from build123d import *

# Parameters (mm, degrees)
F0_R             = 22.25
F1_DEPTH         = 0.8
F2_W             = 8
F2_H             = 8
F3_DEPTH         = 5.7
F4_W             = 8
F4_H             = 6
F5_DEPTH         = 2.9
F6_R             = 0.75
F7_DEPTH         = 0.8
F7_COPIES_COUNT  = 4
F7_COPIES_ANGLE  = 67.5
F7_COPIES1_COUNT = 4
F7_COPIES1_ANGLE = 337.5
F7_COPIES2_COUNT = 3
F7_COPIES2_ANGLE = 315
F7_COPIES3_COUNT = 3
F7_COPIES3_ANGLE = 225
F8_DEPTH         = 0.1
F8_COPIES_COUNT  = 4
F8_COPIES_ANGLE  = 67.5
F8_COPIES1_COUNT = 4
F8_COPIES1_ANGLE = 337.5
F8_COPIES2_COUNT = 3
F8_COPIES2_ANGLE = 315
F8_COPIES3_COUNT = 3
F8_COPIES3_ANGLE = 225


# Not quite as in the source:
# - after a boolean that leaves OpenCascade's solid faulty, fix() repairs it
# - a feature of the source that left no trace in its solid (it failed there, or was rolled back) is left out
# - a pattern or mirror of a feature is missing from the dataset's text; its kind, count and spacing are read off the source's solid


with BuildPart() as f1:
    # F0 (on Top) → F1 (new body)
    with BuildSketch(Plane.XY):
        Circle(F0_R)
    extrude(amount=F1_DEPTH)

    # F2 (on face) → F3 (join)
    with BuildSketch(Plane.XY.offset(0.8)):
        with Locations((0, -17.8874964306)):
            Rectangle(F2_W, F2_H)
    extrude(amount=F3_DEPTH)

    # F4 (on face) → F5 (join)
    with BuildSketch(Plane.XY.offset(0.8)):
        with Locations((0, 18.82292144)):
            Rectangle(F4_W, F4_H)
    extrude(amount=F5_DEPTH)

    # F6 (on face) → F7 (cut, through all)
    with BuildSketch(Plane.XY.offset(0.8)):
        with Locations((-20, 0)):
            Circle(F6_R)
    f7 = extrude(amount=-F7_DEPTH, mode=Mode.SUBTRACT)

    # F7_copies: F7 ×4 about axis
    f7_copies_axis = Axis((0, 0, 0), (0, 0, 1))
    for i in range(1, F7_COPIES_COUNT):
        add(f7.rotate(f7_copies_axis, i * F7_COPIES_ANGLE / (F7_COPIES_COUNT - 1)), mode=Mode.SUBTRACT)

    # F7_copies1: F7 ×4 about axis
    f7_copies1_axis = Axis((0, 0, 0), (0, 0, 1))
    for i in range(1, F7_COPIES1_COUNT):
        add(f7.rotate(f7_copies1_axis, i * F7_COPIES1_ANGLE / (F7_COPIES1_COUNT - 1)), mode=Mode.SUBTRACT)

    # F7_copies2: F7 ×3 about axis
    f7_copies2_axis = Axis((0, 0, 0), (0, 0, 1))
    for i in range(1, F7_COPIES2_COUNT):
        add(f7.rotate(f7_copies2_axis, i * F7_COPIES2_ANGLE / (F7_COPIES2_COUNT - 1)), mode=Mode.SUBTRACT)

    # F7_copies3: F7 ×3 about axis
    f7_copies3_axis = Axis((0, 0, 0), (0, 0, -1))
    for i in range(1, F7_COPIES3_COUNT):
        add(f7.rotate(f7_copies3_axis, i * F7_COPIES3_ANGLE / (F7_COPIES3_COUNT - 1)), mode=Mode.SUBTRACT)

    # F7_copies4: F7 across plane
    add(f7.mirror(Plane(origin=(0, 0, 0), x_dir=(-0.195090322, 0.9807852804, 0), z_dir=(0.9807852804, 0.195090322, 0))), mode=Mode.SUBTRACT)

    # F7_copies5: F7 across plane
    add(f7.mirror(Plane(origin=(0, 0, 0), x_dir=(0.8314696123, -0.555570233, 0), z_dir=(0.555570233, 0.8314696123, 0))), mode=Mode.SUBTRACT)

    # F7_copies6: F7 across plane
    add(f7.mirror(Plane(origin=(0, 0, 0), x_dir=(0, 0, 1), z_dir=(1, 0, 0))), mode=Mode.SUBTRACT)

    # F6 (on face) → F8 (join)
    with BuildSketch(Plane.XY.offset(0.8)):
        with BuildLine():
            Line((-22.0468251683, -3), (-20, -3))
            ThreePointArc((-20, -3), (-17.75, 0), (-20, 3))
            Line((-20, 3), (-22.0468251683, 3))
            ThreePointArc((-22.0468251683, 3), (-22.25, 0), (-22.0468251683, -3))
        make_face()
        with Locations((-20, 0)):
            Circle(F6_R, mode=Mode.SUBTRACT)
    f8 = extrude(amount=F8_DEPTH)

    # F8_copies: F8 ×4 about axis
    f8_copies_axis = Axis((0, 0, 0), (0, 0, 1))
    for i in range(1, F8_COPIES_COUNT):
        add(f8.rotate(f8_copies_axis, i * F8_COPIES_ANGLE / (F8_COPIES_COUNT - 1)))

    # F8_copies1: F8 ×4 about axis
    f8_copies1_axis = Axis((0, 0, 0), (0, 0, 1))
    for i in range(1, F8_COPIES1_COUNT):
        add(f8.rotate(f8_copies1_axis, i * F8_COPIES1_ANGLE / (F8_COPIES1_COUNT - 1)))

    # F8_copies2: F8 ×3 about axis
    f8_copies2_axis = Axis((0, 0, 0), (0, 0, 1))
    for i in range(1, F8_COPIES2_COUNT):
        add(f8.rotate(f8_copies2_axis, i * F8_COPIES2_ANGLE / (F8_COPIES2_COUNT - 1)))

    # F8_copies3: F8 ×3 about axis
    f8_copies3_axis = Axis((0, 0, 0), (0, 0, -1))
    for i in range(1, F8_COPIES3_COUNT):
        add(f8.rotate(f8_copies3_axis, i * F8_COPIES3_ANGLE / (F8_COPIES3_COUNT - 1)))

    # F8_copies4: F8 across plane
    add(f8.mirror(Plane(origin=(0, 0, 0), x_dir=(-0.195090322, 0.9807852804, 0), z_dir=(0.9807852804, 0.195090322, 0))))

    # F8_copies5: F8 across plane
    add(f8.mirror(Plane(origin=(0, 0, 0), x_dir=(0.8314696123, -0.555570233, 0), z_dir=(0.555570233, 0.8314696123, 0))))

    add(f1.part.fix(), mode=Mode.REPLACE)

    # F8_copies6: F8 across plane
    add(f8.mirror(Plane(origin=(0, 0, 0), x_dir=(0, 0, 1), z_dir=(1, 0, 0))))


solid = f1.part
Source: CAD feature listing. Evaluate the final solid. Frame: model axes, mm. A direction names the side the tool comes from. Coordinates: 2 decimals unless noted, no trailing zeros. Order: outer loops, then holes, each group sorted by start corner. A loop starts at its lowest first (then second) coordinate and runs counter-clockwise, first axis right, second up.
Item 1: Pull-direction query (X, two-part tool) for faces 1 (the face through (0, 0, 0)), 2 (the face through (19.202, -7.46, 0.444)); classes: pulls with the +X half, pulls with the -X half, needs draft (parallel to the pull), parting line crosses it, or undercut.
Output values:
face 1: needs draft
face 2: undercut
Item 2: Set-up query: faces 3 (the face through (9, 19, 0.9)), 4 (the face through (0, 19, 3.7)), 5 (the face through (-20.75, 0.03, 0.44)). Return all of +Z, -Z, +X, -X, +Y, -Y with unobstructed straight access to the full face (end or side cutting, diameter ignored); none if empty.
Output values:
face 3: +Z, +X, +Y, -Y
face 4: +Z, +X, -X, +Y
face 5: +Z, -Z
Item 3: Cut plane D-D (z = 5.25). Return loops of the section in (x, y), plus the area to 3 significant figures.
Output values:
outline: (-4, -21.89) - (4, -21.89) - (4, -13.89) - (-4, -13.89) - close
area: 64.0 mm2
Item 4: Cut plane C-C (x = -3). Return loops of the section in (y, z).
Output values:
outline: (-22.05, 0) - (22.05, 0) - (22.05, 0.8) - (21.82, 0.8) - (21.82, 3.7) - (15.82, 3.7) - (15.82, 0.8) - (-13.89, 0.8) - (-13.89, 6.5) - (-21.89, 6.5) - (-21.89, 0.8) - (-22.05, 0.8) - close
Item 5: Material intervals for line 1 (Y direction, x = -0.5, z = 3.5); line 2 (Z direction, x = -7, y = 20.5); line 3 (Z direction, x = 10, y = -6.5), sorted ascending.
Output values:
line 1: y = -21.89 to -13.89, 15.82 to 21.82
line 2: z = 0 to 0.9
line 3: z = 0 to 0.8
Item 6: Cut plane A-A (z = 3). Return loops of the section in (x, y), plus the area to 3 significant figures.
Output values:
outline: (-4, -21.89) - (4, -21.89) - (4, -13.89) - (-4, -13.89) - close; (-4, 15.82) - (4, 15.82) - (4, 21.82) - (-4, 21.82) - close
area: 112 mm2
Item 7: First-contact query: P1, Ø6, axis at x = 19, y = 8.5, coming from the +Z side; P2, Ø5, axis at x = -17, y = -0.5, coming from the -Z side; P3, Ø6, axis at x = -6.5, y = 18.5, coming from the +Z side; P4, Ø2, axis at y = -2.5, z = 1, coming from the -X side. Flat tips, straight axial feed; report the tip coordinate or a pass-through.
Output values:
P1: stops at z = 0.9
P2: stops at z = 0
P3: stops at z = 3.7
P4: stops at x = -22.2
Item 8: Cut plane B-B (y = 0). Return loops of the section in (x, z), plus the area to 3 significant figures.
Output values:
outline: (-22.25, 0) - (-20.75, 0) - (-20.75, 0.9) - (-22.25, 0.9) - close; (-19.25, 0) - (19.25, 0) - (19.25, 0.9) - (17.75, 0.9) - (17.75, 0.8) - (-17.75, 0.8) - (-17.75, 0.9) - (-19.25, 0.9) - close; (20.75, 0) - (22.25, 0) - (22.25, 0.9) - (20.75, 0.9) - close
area: 33.8 mm2
